Input: part model. Units: mm. Frame: model coordinates. A direction names the side the tool comes from. Round coordinates to 2 decimals unless told otherwise and drop trailing zeros. Loops run counter-clockwise (first coordinate to the right, second up) from the corner with the lowest first, then second, coordinate; pieces in that order, holes last. Notation, with made-up numbers: (2.25, -34.5) - (6.25, -34.5) arc R28 ccw to (6.25, -6.5) - close; hole circle Ø4 at (-24, 29). An arc over 180 degrees is marked (long way). One line per question, with ' | ' between items. Start each with the question number.
Item 1: Section B-B, the plane x = 29. Return loops of the section in (y, z).
Item 2: First-contact query: pin 1 (1 mm diameter, centred on x = 22.5, z = 6, fed in from +Y); pin 2 (4 mm diameter, centred on y = 2.5, z = 5, fed in from -X); pin 3 (4 mm diameter, centred on x = -6.5, z = 5.5, fed in from -Y); pin 4 (10.5 mm diameter, centred on x = 13, y = 3.5, fed in from +Z). Flat tips, straight axial feed; report the tip coordinate or a pass-through.
Item 3: Section C-C, the plane z = 5. Return loops of the section in (x, y).
Item 4: Material intervals for line 1 along Y through (x, z) = (13.5, 5.5); line 2 along X through (y, z) = (12, 3.25); line 3 along Y through (x, z) = (8.5, 2.25), sorted ascending.
Item 5: Section A-A, the plane y = 6.5. Return loops of the section in (x, z), plus the area to 3 significant figures.
Item 6: Draft query along Y for faces 6 (the face through (0, 15, 5)), 7 (the face through (-3, -14, 7.5)), 8 (the face through (0, -13.5, 4)), 9 (the face through (0, -15, 5)). Return one class per face: pulls with the +Y half, pulls with the -Y half, needs draft (parallel to the pull), parting line crosses it, or undercut.
Item 7: Set-up query: faces 1 (the face through (-31, 0, 4)), 2 (the face through (35, 0, 1)), 3 (the face through (0, 17.5, 1)), 4 (the face through (32.5, 0, 5)), 5 (the face through (-32.5, 0, 5)). Return all of +Z, -Z, +X, -X, +Y, -Y with unobstructed straight access to the full face (end or side cutting, diameter ignored); none if empty.
Item 8: Section D-D, the plane z = 1. Return loops of the section in (x, y), plus the area to 3 significant figures.
```python
from build123d import *

# Parameters (mm, degrees)
F0_W     = 70
F0_H     = 35
F1_DEPTH = 2.5
F2_W     = 65
F2_H     = 30
F2_W_2   = 62
F2_H_2   = 27
F3_DEPTH = 5
F4_DEPTH = 2.5


# Not quite as in the source:
# - the program builds the solid bodies; features that only make, move or delete a surface that nothing else refers to are left out


with BuildPart() as f1:
    # F0 (on Top) → F1 (new body)
    with BuildSketch(Plane.XY):
        Rectangle(F0_W, F0_H)
    extrude(amount=F1_DEPTH)

    # F2 (on face) → F3 (join)
    with BuildSketch(Plane.XY.offset(2.5)):
        Rectangle(F2_W, F2_H)
        Rectangle(F2_W_2, F2_H_2, mode=Mode.SUBTRACT)
    extrude(amount=F3_DEPTH)

    # F4 (cut, through all): a face of the model
    f4_faces = [f1.faces().sort_by_distance(p)[0] for p in [
        (0, 0, 2.5),
    ]]
    extrude(f4_faces, amount=-F4_DEPTH, mode=Mode.SUBTRACT)


solid = f1.part
```
Return value:
1) outline: (-17.5, 0) - (-13.5, 0) - (-13.5, 7.5) - (-15, 7.5) - (-15, 2.5) - (-17.5, 2.5) - close; (13.5, 0) - (17.5, 0) - (17.5, 2.5) - (15, 2.5) - (15, 7.5) - (13.5, 7.5) - close
2) pin 1: y = 15 | pin 2: x = -32.5 | pin 3: y = -15 | pin 4: through
3) outline: (-32.5, -15) - (32.5, -15) - (32.5, 15) - (-32.5, 15) - close; hole (-31, -13.5) - (31, -13.5) - (31, 13.5) - (-31, 13.5) - close
4) line 1: -15 to -13.5, 13.5 to 15 | line 2: -32.5 to -31, 31 to 32.5 | line 3: -17.5 to -13.5, 13.5 to 17.5
5) outline: (-35, 0) - (-31, 0) - (-31, 7.5) - (-32.5, 7.5) - (-32.5, 2.5) - (-35, 2.5) - close; (31, 0) - (35, 0) - (35, 2.5) - (32.5, 2.5) - (32.5, 7.5) - (31, 7.5) - close | area: 35.0 mm2
6) face 6: pulls with the +Y half | face 7: needs draft | face 8: undercut | face 9: pulls with the -Y half
7) face 1: +Z, -Z | face 2: +Z, -Z, +X, +Y, -Y | face 3: +Z, -Z, +X, -X, +Y | face 4: +Z, +X, +Y, -Y | face 5: +Z, -X, +Y, -Y
8) outline: (-35, -17.5) - (35, -17.5) - (35, 17.5) - (-35, 17.5) - close; hole (-31, -13.5) - (31, -13.5) - (31, 13.5) - (-31, 13.5) - close | area: 776 mm2
